from build123d import *

# Parameters (mm, degrees)
SKETCH2_W           = 270
SKETCH2_H           = 225
BOSS_EXTRUDE1_DEPTH = 10
BOSS_EXTRUDE4_DEPTH = 270
SKETCH5_W           = 64.951905284
SKETCH5_H           = 10
CUT_EXTRUDE1_DEPTH  = 302.95039014
SKETCH6_W           = 64.951905284
SKETCH6_H           = 10
CUT_EXTRUDE2_DEPTH  = 302.95039014
SKETCH7_W           = 64.951905284
SKETCH7_H           = 10
CUT_EXTRUDE3_DEPTH  = 302.95039014


with BuildPart() as part:
    # Sketch2 → Boss-Extrude1 (new body)
    with BuildSketch(Plane(origin=(0, 0, 0), x_dir=(0, 0, -1), z_dir=(1, 0, 0))):
        with Locations((135, 112.5)):
            Rectangle(SKETCH2_W, SKETCH2_H)
    extrude(amount=BOSS_EXTRUDE1_DEPTH)

    # Sketch4 → Boss-Extrude4 (add)
    with BuildSketch(Plane.XY):
        Polygon((10, 225), (74.951905284, 112.5), (10, 112.5), align=None)
    extrude(amount=-BOSS_EXTRUDE4_DEPTH)

    # Sketch5 → Cut-Extrude1 (cut, through all)
    with BuildSketch(Plane.XZ.offset(-112.5)):
        with Locations((42.475952642, -265)):
            Rectangle(SKETCH5_W, SKETCH5_H)
    extrude(amount=-CUT_EXTRUDE1_DEPTH, mode=Mode.SUBTRACT)

    # Sketch6 → Cut-Extrude2 (cut, through all)
    with BuildSketch(Plane.XZ.offset(-112.5)):
        with Locations((42.475952642, -245)):
            Rectangle(SKETCH6_W, SKETCH6_H)
    extrude(amount=-CUT_EXTRUDE2_DEPTH, mode=Mode.SUBTRACT)

    # Sketch7 → Cut-Extrude3 (cut, through all)
    with BuildSketch(Plane.XZ.offset(-112.5)):
        with Locations((42.475952642, -5)):
            Rectangle(SKETCH7_W, SKETCH7_H)
        with Locations((42.475952642, -25)):
            Rectangle(SKETCH7_W, SKETCH7_H)
        with Locations((42.475952642, -45)):
            Rectangle(SKETCH7_W, SKETCH7_H)
        with Locations((42.475952642, -65)):
            Rectangle(SKETCH7_W, SKETCH7_H)
        with Locations((42.475952642, -85)):
            Rectangle(SKETCH7_W, SKETCH7_H)
        with Locations((42.475952642, -105)):
            Rectangle(SKETCH7_W, SKETCH7_H)
        with Locations((42.475952642, -125)):
            Rectangle(SKETCH7_W, SKETCH7_H)
        with Locations((42.475952642, -145)):
            Rectangle(SKETCH7_W, SKETCH7_H)
        with Locations((42.475952642, -165)):
            Rectangle(SKETCH7_W, SKETCH7_H)
        with Locations((42.475952642, -185)):
            Rectangle(SKETCH7_W, SKETCH7_H)
        with Locations((42.475952642, -205)):
            Rectangle(SKETCH7_W, SKETCH7_H)
        with Locations((42.475952642, -225)):
            Rectangle(SKETCH7_W, SKETCH7_H)
    extrude(amount=-CUT_EXTRUDE3_DEPTH, mode=Mode.SUBTRACT)


solid = part.part
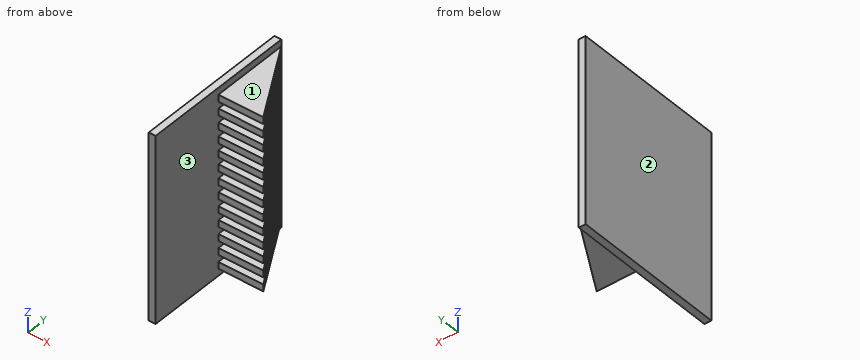
Source: CAD feature listing. Evaluate the final solid. Frame: model axes, mm. Face numbers are marked on the shaded views. Round coordinates to 2 decimals unless told otherwise and drop trailing zeros. Loops run counter-clockwise (first coordinate to the right, second up) from the corner with the lowest first, then second, coordinate; pieces in that order, holes last. Notation, with made-up numbers: (-14.5, 40) -> (33.5, 40) arc R19 ccw to (33.5, 75) -> close; hole circle Ø2 at (-13.5, -38.75). An arc over 180 degrees is marked (long way). Answer as a JSON object with one key per item and string values. Group by question number.
Q1. Mould query, pull axis Z, two halves, no side actions, for the marked faces 1, 2 and 3. Classes: pulls with the +Z half, pulls with the -Z half, needs draft (parallel to the pull), parting line crosses it, or undercut.
Q2. Section query A-A (z = -175). Output: boundary loops of the cut face in (x, y).
Q3. Section query B-B (x = 48.5). State how many separate pieces and enclosed holes the cut face has, plus the area to 3 significant figures.
Q4. Contact query for flat-ended pins moving along their axis: P1, Ø8, axis at x = 43.5, z = -236, coming from the -Y side; P2, Ø19.5, axis at x = 27.5, y = 171, coming from the +Z side; P3, Ø19.5, axis at x = 35, y = 184.5, coming from the -Z side. Output: stop coordinate, or through.
Q5. Ray query, line 1 (X direction, y = 148.5, z = -189.5); line 2 (Y direction, x = 40, z = -95); line 3 (Y direction, x = 28, z = -193). Return the intervals inside material, ascending. Write a range as from..to.
Q6. Section query C-C (y = 53.5). Output: boundary loops of the cut face in (x, z), plus the area to 3 significant figures.
Completed:
{
 "1": {"face 1": "pulls with the +Z half", "face 2": "needs draft", "face 3": "undercut"},
 "2": {"outline": "(0, 0) -> (10, 0) -> (10, 112.5) -> (74.95, 112.5) -> (10, 225) -> (0, 225) -> close"},
 "3": {"separate pieces": "13", "enclosed holes": "0", "area": "5,960 mm²"},
 "4": {"P1": "y = 112.5", "P2": "z = -10", "P3": "z = -260"},
 "5": {"line 1": "0..10", "line 2": "112.5..173.04", "line 3": "112.5..193.82"},
 "6": {"outline": "(0, -270) -> (10, -270) -> (10, 0) -> (0, 0) -> close", "area": "2,700 mm²"}
}
